Autodesk Inventor part; units mm, degrees
ref_plane "YZ Plane" through (0, 0, 0) normal (1, 0, 0) x (0, 1, 0)
ref_plane "XZ Plane" through (0, 0, 0) normal (0, 1, 0) x (-1, 0, 0)
ref_plane "XY Plane" through (0, 0, 0) normal (0, 0, 1) x (1, 0, 0)
sketch "Sketch1" plane through (0, 0, 0) normal (0, 0, 1) x (1, 0, 0)
  circle A0 centre (0, 0) radius 31
  dimension "d0" = 62
extrude "Extrusion1" add sketch "Sketch1" along normal blind 100
chamfer "Chamfer1" distance 2 angle 45 2 edges at (-31, 0, 100) (-31, 0, 0)
sketch "Sketch2" plane through (0, 0, 100) normal (0, 0, 1) x (1, 0, 0)
  circle A0 centre (0, 0) radius 15.5
  dimension "d6" = 31
extrude "Extrusion2" add sketch "Sketch2" along normal blind 100
fillet "Fillet1" radius 2 1 edges at (-15.5, 0, 200)
fillet "Fillet2" radius 2 1 edges at (-15.5, 0, 100)
sketch "Sketch3" plane through (0, 0, 0) normal (0, 0, -1) x (-1, 0, 0)
  circle A0 centre (0, 0) radius 31
  dimension "d11" = 62
extrude "Extrusion3" cut sketch "Sketch3" against normal blind 30
fillet "Fillet3" radius 2 1 edges at (-31, 0, 30)
properties part number "S.motor"
For this review, take the finished solid that the model builds, in its own axes (mm). A direction names the side the tool comes from. Round coordinates to 2 decimals unless told otherwise and drop trailing zeros. Write each loop counter-clockwise with the first axis right and the second up, starting at its lowest first coordinate (ties: lowest second). Pieces come first, ordered by that corner, then holes. Notation, with made-up numbers: (16, 71) - (56, 71) arc R21 cw to (56, 97) - close; hole circle Ø2 at (-14.5, 31.5). An arc over 180 degrees is marked (long way). Write item = value, one per line. Start each with the question number.
1. For faces 1 (the face through (0, 0, 200)), 2 (the face through (12.5, -12.5, 100)), list the 3-axis set-ups (+Z, -Z, +X, -X, +Y, -Y) from which the entire face can be reached by the end or side of a thin tool; tool diameter is ignored.
2. Consider section A-A on y = 0. State the section outline as (x, z) points.
3. Consider section C-C on z = 133. State the section outline as (x, y) points.
4. Consider section D-D on z = 93.5. State the section outline as (x, y) points, plus the area to 3 significant figures.
5. For pin 1 Ø12 at (x, z) = (-4, 180.5) entering from +Y; pin 2 Ø1.5 at (x, y) = (-11.5, 16) entering from +Z; pin 3 Ø12 at (x, y) = (20.5, -0.5) entering from +Z; pin 4 Ø8 at (x, y) = (2.5, 16.5) entering from +Z, all flat-tipped, find the tip position at first contact; note any pin that passes through.
6. Wall thickness on L1, parallel to Z at x = 14, y = 16; L2, parallel to Z at x = -10.5, y = 9; L3, parallel to Y at x = 27, z = 73: over which ranges is each line inside the solid? List them lowest first.
Evaluation:
q1.face_1 = +Z, +X, -X, +Y, -Y
q1.face_2 = +Z
q2.outline = (-31, 32) arc R2 ccw to (-29, 30) - (29, 30) arc R2 ccw to (31, 32) - (31, 98) - (29, 100) - (17.5, 100) arc R2 cw to (15.5, 102) - (15.5, 198) arc R2 ccw to (13.5, 200) - (-13.5, 200) arc R2 ccw to (-15.5, 198) - (-15.5, 102) arc R2 cw to (-17.5, 100) - (-29, 100) - (-31, 98) - close
q3.outline = circle Ø31 at (0, 0)
q4.outline = circle Ø62 at (0, 0)
q4.area = 3,020 mm2
q5.pin_1 = 15.5
q5.pin_2 = 100
q5.pin_3 = 199.73
q5.pin_4 = 200
q6.L1 = 30 to 100
q6.L2 = 30 to 199.97
q6.L3 = -15.23 to 15.23
